For this review, take the finished solid that the model builds, in its own axes (mm). Give positions to 0.01 mm unless a question says otherwise; leave off trailing zeros. Loops run counter-clockwise (first coordinate to the right, second up) from the corner with the lowest first, then second, coordinate; pieces in that order, holes last.
Autodesk Inventor part; units mm, degrees
ref_plane "YZ Plane" through (0, 0, 0) normal (1, 0, 0) x (0, 1, 0)
ref_plane "XZ Plane" through (0, 0, 0) normal (0, 1, 0) x (-1, 0, 0)
ref_plane "XY Plane" through (0, 0, 0) normal (0, 0, 1) x (1, 0, 0)
sketch "Эскиз1" plane through (0, 0, 0) normal (0, 1, 0) x (-1, 0, 0)
  line L0 (-30, -72.5) -> (30, -72.5)
  line L1 (30, -72.5) -> (30, 72.5)
  line L2 (30, 72.5) -> (-30, 72.5)
  line L3 (-30, 72.5) -> (-30, -72.5)
  line L4 (-30, -72.5) -> (30, 72.5) construction
  line L5 (30, -72.5) -> (-30, 72.5) construction
  point P0 (0, 0)
  dimension "d0" = 145
  dimension "d1" = 60
extrude "Выдавливание1" add sketch "Эскиз1" along normal mid plane 6
sketch "Эскиз2" plane through (0, 3, 0) normal (0, 1, 0) x (1, 0, 0)
  circle A0 centre (15, -42.0468) radius 2.1
  circle A1 centre (15, 33.9532) radius 2.6
  point P0 (0, 0)
extrude "Выдавливание2" cut sketch "Эскиз2" against normal up to next
properties part number "проставка"
Q1. For probe 1 along Z at (x, y) = (15, 0.8), list the stretches that pass through material, from the lowest coordinate up.
Answers:
probe 1: z = -72.5 to -36.55, -31.35 to 39.95, 44.15 to 72.5
Q2. Mouldability with a two-part tool opening along Z and no side actions: class faces 1 (the flat face through (-30, 0, -1)), 2 (the cylindrical face through (14.545, 0.042, 44.097)), 3 (the flat face through (0, 0, -72.5)) as +Z half, -Z half, draft (parallel to the pull), parting line (faces both ways), or undercut.
Answers:
face 1: draft
face 2: undercut
face 3: -Z half
Q3. Consider section A-A on x = 15. Give the boundary of the cut face in (y, z), plus the area to 3 significant figures.
Answers:
outline: (-3, -72.5) - (3, -72.5) - (3, -36.55) - (-3, -36.55) - close; (-3, -31.35) - (3, -31.35) - (3, 39.95) - (-3, 39.95) - close; (-3, 44.15) - (3, 44.15) - (3, 72.5) - (-3, 72.5) - close
area: 814 mm2
